Here's how the part is built. I have some questions about the finished solid (model axes, mm). Face numbers are marked on the shaded views. A direction names the side the tool comes from. Round coordinates to 2 decimals unless told otherwise and drop trailing zeros. Write each loop counter-clockwise with the first axis right and the second up, starting at its lowest first coordinate (ties: lowest second). Pieces come first, ordered by that corner, then holes. Notation, with made-up numbers: (-2, 5.25) -> (36, 5.25) arc R22 ccw to (36, 26.25) -> close; hole circle Ø9 at (7, 16.5). An arc over 180 degrees is marked (long way). Answer in a Markdown table with one row per item.
from build123d import *

# Parameters (mm, degrees)
F0_W     = 69.85
F0_H     = 44.45
F1_DEPTH = 38.1
F3_DEPTH = 38.101
F4_DEPTH = 25.4
F5_R     = 3.175
F6_DEPTH = 6.351
F8_DEPTH = 12.701


with BuildPart() as f1:
    # F0 (on Front) → F1 (new body)
    with BuildSketch(Plane.XZ):
        with Locations((-14.4096150837, 22.225)):
            Rectangle(F0_W, F0_H)
    extrude(amount=F1_DEPTH)

    # F2 (on face) → F3 (cut, through all)
    with BuildSketch(Plane.XZ.offset(38.1)):
        with BuildLine():
            Line((-49.3346150837, 44.45), (-49.3346150837, 31.75))
            ThreePointArc((-49.3346150837, 31.75), (-45.6148712048, 40.7302561211), (-36.6346150837, 44.45))
            Line((-36.6346150837, 44.45), (-49.3346150837, 44.45))
        make_face()
        with BuildLine():
            Line((-23.9346150837, 31.75), (-23.9346150837, 19.05))
            Line((-23.9346150837, 19.05), (1.4653849163, 19.05))
            Line((1.4653849163, 19.05), (20.5153849163, 19.05))
            Line((20.5153849163, 19.05), (20.5153849163, 44.45))
            Line((20.5153849163, 44.45), (-36.6346150837, 44.45))
            ThreePointArc((-36.6346150837, 44.45), (-27.6543589626, 40.7302561211), (-23.9346150837, 31.75))
        make_face()
        with BuildLine():
            Line((1.4653849163, 19.05), (-23.9346150837, 19.05))
            ThreePointArc((-23.9346150837, 19.05), (-20.2148712048, 10.0697438789), (-11.2346150837, 6.35))
            ThreePointArc((-11.2346150837, 6.35), (-2.2543589626, 10.0697438789), (1.4653849163, 19.05))
        make_face()
        with BuildLine():
            Line((-11.2346150837, 6.35), (20.5153849163, 6.35))
            Line((20.5153849163, 6.35), (20.5153849163, 19.05))
            Line((20.5153849163, 19.05), (1.4653849163, 19.05))
            ThreePointArc((1.4653849163, 19.05), (-2.2543589626, 10.0697438789), (-11.2346150837, 6.35))
        make_face()
    extrude(amount=-F3_DEPTH, mode=Mode.SUBTRACT)

    # F2 (on face) → F4 (cut)
    with BuildSketch(Plane.XZ.offset(38.1)):
        Polygon((-49.3346150837, 31.75), (-49.3346150837, 6.35), (-23.9346150837, 6.35), (-23.9346150837, 19.05), (-23.9346150837, 31.75), align=None)
        with BuildLine():
            Line((-23.9346150837, 19.05), (-23.9346150837, 6.35))
            Line((-23.9346150837, 6.35), (-11.2346150837, 6.35))
            ThreePointArc((-11.2346150837, 6.35), (-20.2148712048, 10.0697438789), (-23.9346150837, 19.05))
        make_face()
        with BuildLine():
            ThreePointArc((-23.9346150837, 31.75), (-36.6346150837, 44.45), (-49.3346150837, 31.75))
            Line((-49.3346150837, 31.75), (-23.9346150837, 31.75))
        make_face()
        with BuildLine():
            Line((1.4653849163, 19.05), (-23.9346150837, 19.05))
            ThreePointArc((-23.9346150837, 19.05), (-20.2148712048, 10.0697438789), (-11.2346150837, 6.35))
            ThreePointArc((-11.2346150837, 6.35), (-2.2543589626, 10.0697438789), (1.4653849163, 19.05))
        make_face()
        with BuildLine():
            ThreePointArc((1.4653849163, 19.05), (-2.2543589626, 10.0697438789), (-11.2346150837, 6.35))
            Line((-11.2346150837, 6.35), (20.5153849163, 6.35))
            Line((20.5153849163, 6.35), (20.5153849163, 19.05))
            Line((20.5153849163, 19.05), (1.4653849163, 19.05))
        make_face()
    extrude(amount=-F4_DEPTH, mode=Mode.SUBTRACT)

    # F5 (on face) → F6 (cut, through all)
    with BuildSketch(Plane.XY.offset(6.35)):
        with Locations((10.9903849163, -8.5281981155)):
            Circle(F5_R)
        with Locations((10.9903849163, -28.575)):
            Circle(F5_R)
        with BuildLine():
            ThreePointArc((-42.9846150837, -38.1), (-47.4747431442, -36.2401280605), (-49.3346150837, -31.75))
            Line((-49.3346150837, -31.75), (-49.3346150837, -38.1))
            Line((-49.3346150837, -38.1), (-42.9846150837, -38.1))
        make_face()
        with BuildLine():
            ThreePointArc((20.5153849163, -31.75), (18.6555129768, -36.2401280605), (14.1653849163, -38.1))
            Line((14.1653849163, -38.1), (20.5153849163, -38.1))
            Line((20.5153849163, -38.1), (20.5153849163, -31.75))
        make_face()
        with Locations((-36.6346150837, -28.575)):
            Circle(F5_R)
    extrude(amount=-F6_DEPTH, mode=Mode.SUBTRACT)

    # F7 (on face) → F8 (cut, through all)
    with BuildSketch(Plane.XZ.offset(12.7)):
        with BuildLine():
            Line((-36.6346150837, 31.75), (-36.6346150837, 38.1))
            ThreePointArc((-36.6346150837, 38.1), (-41.1247431442, 36.2401280605), (-42.9846150837, 31.75))
            Line((-42.9846150837, 31.75), (-36.6346150837, 31.75))
        make_face()
        with BuildLine():
            ThreePointArc((-30.2846150837, 31.75), (-32.1444870232, 36.2401280605), (-36.6346150837, 38.1))
            Line((-36.6346150837, 38.1), (-36.6346150837, 31.75))
            Line((-36.6346150837, 31.75), (-30.2846150837, 31.75))
        make_face()
        with BuildLine():
            Line((-30.2846150837, 31.75), (-36.6346150837, 31.75))
            Line((-36.6346150837, 31.75), (-36.6346150837, 25.4))
            ThreePointArc((-36.6346150837, 25.4), (-32.1444870232, 27.2598719395), (-30.2846150837, 31.75))
        make_face()
        with BuildLine():
            Line((-36.6346150837, 25.4), (-36.6346150837, 31.75))
            Line((-36.6346150837, 31.75), (-42.9846150837, 31.75))
            ThreePointArc((-42.9846150837, 31.75), (-41.1247431442, 27.2598719395), (-36.6346150837, 25.4))
        make_face()
    extrude(amount=-F8_DEPTH, mode=Mode.SUBTRACT)


solid = f1.part
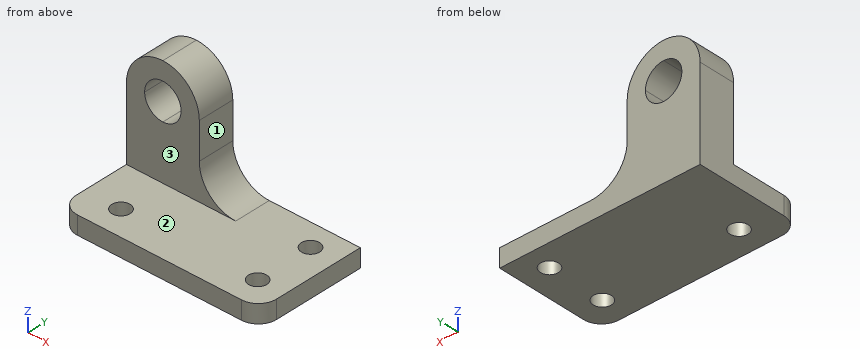
1) I want a section at B-B, the plane z = 27.5. List the corners of the cut face in (x, y) for me.
Response:
| item | result |
|---|---|
| outline | (-49.33, -12.7) -> (-41.35, -12.7) -> (-41.35, 0) -> (-49.33, 0) -> close; (-31.92, -12.7) -> (-23.93, -12.7) -> (-23.93, 0) -> (-31.92, 0) -> close |
2) I want a section at A-A, the plane y = -7.5. List the corners of the cut face in (x, z) for me, and give its area (3 significant figures).
Response:
| item | result |
|---|---|
| outline | (-49.33, 0) -> (7.99, 0) -> (7.99, 6.35) -> (-11.23, 6.35) arc R12.7 cw to (-23.93, 19.05) -> (-23.93, 31.75) arc R12.7 ccw to (-49.33, 31.75) -> close; (13.99, 0) -> (20.52, 0) -> (20.52, 6.35) -> (13.99, 6.35) -> close; hole circle Ø12.7 at (-36.63, 31.75) |
| area | 1,210 mm^2 |
3) For pin 1 (10 mm diameter, centred on y = -6.5, z = 25.5, fed in from +X); pin 2 (6 mm diameter, centred on x = -23, z = 19.5, fed in from -Y); pin 3 (6 mm diameter, centred on x = -38.5, y = -21, fed in from +Z), each with a flat end and sliding along its axis, tell me the tip position at first contact or that it passes through.
Response:
| item | result |
|---|---|
| pin 1 | stops at x = -23.93 |
| pin 2 | stops at y = -12.7 |
| pin 3 | stops at z = 6.35 |
4) I want a section at C-C, the plane z = 22.5. List the corners of the cut face in (x, y) for me, and give its area (3 significant figures).
Response:
| item | result |
|---|---|
| outline | (-49.33, -12.7) -> (-23.93, -12.7) -> (-23.93, 0) -> (-49.33, 0) -> close |
| area | 323 mm^2 |
5) I need wall thicknesses on line 1 (Z direction, x = 6.5, y = -10.5); line 2 (X direction, y = -8, z = 24); line 3 (X direction, y = -8.5, z = 31). Which ranges of each line are inside material? Lowest first, please. Write a range as [from, to].
Response:
| item | result |
|---|---|
| line 1 | z = [0, 6.35] |
| line 2 | x = [-49.33, -23.93] |
| line 3 | x = [-49.33, -42.94], [-30.33, -23.93] |
6) Which directions (+Z, -Z, +X, -X, +Y, -Y) give clear straight access to the entire face, cutting with the end or side of a thin tool? Please do the marked faces 1, 2 and 3.
Response:
| item | result |
|---|---|
| face 1 | +Z, +X, +Y, -Y |
| face 2 | +Z, +X, -Y |
| face 3 | +Z, +X, -X, -Y |
